For this review, take the finished solid that the model builds, in its own axes (mm). Face numbers are marked on the shaded views. A direction names the side the tool comes from. Round coordinates to 2 decimals unless told otherwise and drop trailing zeros. Write each loop counter-clockwise with the first axis right and the second up, starting at its lowest first coordinate (ties: lowest second). Pieces come first, ordered by that corner, then holes.
from build123d import *

# Parameters (mm, degrees)
ESQUISSE1_W             = 72
ESQUISSE1_H             = 110
BOSS_EXTRU_1_DEPTH      = 30
D_GAGEMENT_M31_D        = 3.6
ESQUISSE5_W             = 10
ESQUISSE5_H             = 15
ESQUISSE5_W_2           = 38
ENL_V_MAT_EXTRU_1_DEPTH = 30
ESQUISSE6_W             = 28
ESQUISSE6_H             = 15
ESQUISSE6_W_2           = 9
ENL_V_MAT_EXTRU_2_DEPTH = 30


with BuildPart() as part:
    # Esquisse1 → Boss.-Extru.1 (new body)
    with BuildSketch(Plane.XY):
        with Locations((36, 55)):
            Rectangle(ESQUISSE1_W, ESQUISSE1_H)
    extrude(amount=BOSS_EXTRU_1_DEPTH)

    # Dégagement M31 (through all)
    with Locations(Plane.XY.offset(30)):
        with Locations((4, 91), (68, 91), (4, 19), (68, 19)):
            Hole(D_GAGEMENT_M31_D / 2)

    # Esquisse5 → Enlèv. mat.-Extru.1 (cut)
    with BuildSketch(Plane(origin=(0, 0, 0), x_dir=(-1, 0, 0), z_dir=(0, 0, -1))):
        with Locations((-5, 102.5)):
            Rectangle(ESQUISSE5_W, ESQUISSE5_H)
        with Locations((-19, 7.5)):
            Rectangle(ESQUISSE5_W_2, ESQUISSE5_H)
    extrude(amount=-ENL_V_MAT_EXTRU_1_DEPTH, mode=Mode.SUBTRACT)

    # Esquisse6 → Enlèv. mat.-Extru.2 (cut)
    with BuildSketch(Plane(origin=(0, 0, 0), x_dir=(-1, 0, 0), z_dir=(0, 0, -1))):
        with Locations((-58, 102.5)):
            Rectangle(ESQUISSE6_W, ESQUISSE6_H)
        with Locations((-67.5, 7.5)):
            Rectangle(ESQUISSE6_W_2, ESQUISSE6_H)
    extrude(amount=-ENL_V_MAT_EXTRU_2_DEPTH, mode=Mode.SUBTRACT)


solid = part.part
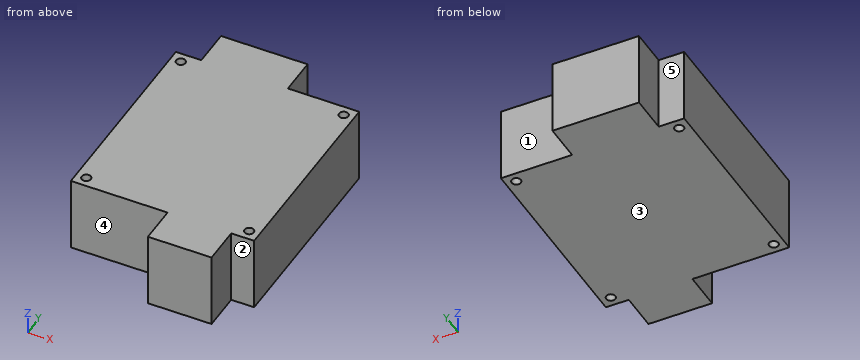
(1) We need section B-B, the plane z = 26.75. Give the boundary of the cut face in (x, y).
Geometry check:
outline: (0, 15) - (38, 15) - (38, 0) - (63, 0) - (63, 15) - (72, 15) - (72, 95) - (44, 95) - (44, 110) - (10, 110) - (10, 95) - (0, 95) - close; hole circle Ø3.6 at (4, 19); hole circle Ø3.6 at (4, 91); hole circle Ø3.6 at (68, 19); hole circle Ø3.6 at (68, 91)
(2) We need section A-A, the plane x = 68. Give the boundary of the cut face in (y, z).
Geometry check:
outline: (15, 0) - (17.2, 0) - (17.2, 30) - (15, 30) - close; (20.8, 0) - (89.2, 0) - (89.2, 30) - (20.8, 30) - close; (92.8, 0) - (95, 0) - (95, 30) - (92.8, 30) - close
(3) For the marked faces 1, 2, 3, 4 and 5, list the 3-axis set-ups (+Z, -Z, +X, -X, +Y, -Y) from which the entire face can be reached by the end or side of a thin tool; tool diameter is ignored.
Geometry check:
face 1: +Z, -Z, +X, +Y
face 2: +Z, -Z, +X, -Y
face 3: -Z, +X, -X, +Y, -Y
face 4: +Z, -Z, -X, -Y
face 5: +Z, -Z, -X, +Y
(4) We need section D-D, the plane x = 48. Give the boundary of the cut face in (y, z), and give its area (3 significant figures).
Geometry check:
outline: (0, 0) - (95, 0) - (95, 30) - (0, 30) - close
area: 2,850 mm2
(5) For pin 1 Ø16.5 at (y, z) = (4.5, 10) entering from +X; pin 2 Ø3 at (x, y) = (4, 19) entering from +Z; pin 3 Ø3 at (x, z) = (53.5, 21) entering from +Y; pin 4 Ø16.5 at (y, z) = (4, 13) entering from -X, all flat-tipped, find the tip position at first contact; note any pin that passes through.
Geometry check:
pin 1: stops at x = 63
pin 2: passes through
pin 3: stops at y = 95
pin 4: stops at x = 38
(6) For line 1 along Y through (x, z) = (68, 7.25); line 2 along Y through (x, z) = (19.5, 12); line 3 along X through (y, z) = (7, 8.75), list the stretches that pass through material, from the lowest coordinate up.
Geometry check:
line 1: y = 15 to 17.2, 20.8 to 89.2, 92.8 to 95
line 2: y = 15 to 110
line 3: x = 38 to 63
(7) We need section C-C, the plane y = 91. Give the boundary of the cut face in (x, z), and give its area (3 significant figures).
Geometry check:
outline: (0, 0) - (2.2, 0) - (2.2, 30) - (0, 30) - close; (5.8, 0) - (66.2, 0) - (66.2, 30) - (5.8, 30) - close; (69.8, 0) - (72, 0) - (72, 30) - (69.8, 30) - close
area: 1,940 mm2
